from build123d import *

# Parameters (mm, degrees)
F0_R     = 30
F0_R_2   = 6.25
F1_DEPTH = 29
F2_R     = 35
F2_R_2   = 6.25
F3_DEPTH = 6
F4_SIZE  = 3


with BuildPart() as f1:
    # F0 (on Top) → F1 (new body)
    with BuildSketch(Plane.XY):
        Circle(F0_R)
        Circle(F0_R_2, mode=Mode.SUBTRACT)
    extrude(amount=F1_DEPTH)

    # F2 (on Top) → F3 (join)
    with BuildSketch(Plane.XY):
        Circle(F2_R)
        Circle(F2_R_2, mode=Mode.SUBTRACT)
    extrude(amount=F3_DEPTH)

    # F4
    f4_edges = [f1.edges().sort_by_distance(p)[0] for p in [
        (-30, 0, 29),
    ]]
    chamfer(f4_edges, length=F4_SIZE)


solid = f1.part
Read the model definition and answer for the solid it produces. Units are mm, in the model's axes. A direction names the side the tool comes from. Give positions to 0.01 mm unless a question says otherwise; leave off trailing zeros. Write each loop counter-clockwise with the first axis right and the second up, starting at its lowest first coordinate (ties: lowest second). Pieces come first, ordered by that corner, then holes. Notation, with made-up numbers: (-20, -28) -> (8, -28) arc R19 ccw to (8, 1) -> close; hole circle Ø7 at (-3, -8). An arc over 180 degrees is marked (long way). Answer as a JSON object with one key per item and string values. Group by question number.
1) Consider L1, parallel to Y at x = 0, z = 19.25; L2, parallel to Z at x = 25, y = -23.5; L3, parallel to X at y = 5, z = 15.25. Determine where each line is inside the solid, lowest interval first. Write a range as from..to.
2) Find section C-C (z = 27). Write down the section's boundary in (x, y).
3) Find section A-A (x = 0). Write down the section's boundary in (y, z), and give its area (3 significant figures).
4) Each of these flat-tipped pins is pushed along its axis until it touches: P1, Ø1, axis at x = 20.5, z = 20.5, coming from the +Y side; P2, Ø1.5, axis at x = 13.5, y = 26, coming from the +Z side; P3, Ø2, axis at x = 0, z = 17.5, coming from the +Y side; P4, Ø20, axis at x = 0, y = 0, coming from the +Z side. Where does it stop, or does it pass through?
5) A tool of negligible diameter and unlimited length cuts with its end or side. For faces 1 (the cylindrical face through (-29.97, 1.32, 15.86)), 2 (the cylindrical face through (-28, -21, 3)), from which of +Z, -Z, +X, -X, +Y, -Y can it reach the whole face along a straight path? Write none if from no direction.
6) The mould has two halves that part along Y. Classify faces 3 (the cylindrical face through (5.96, 1.88, 14.3)), 4 (the conical face through (-3.534, 26.915, 28.854)), 5 (the flat face through (0, -7, 0)): +Y half, -Y half, draft (parallel to the pull), parting line (faces both ways), or undercut.
7) Find section D-D (z = 18). Write down the section's boundary in (x, y), and give its area (3 significant figures).
Values follow:
{
 "1": {"L1": "y = -30..-6.25, 6.25..30", "L2": "z = 0..6", "L3": "x = -29.58..-3.75, 3.75..29.58"},
 "2": {"outline": "circle Ø58 at (0, 0); hole circle Ø12.5 at (0, 0)"},
 "3": {"outline": "(-35, 0) -> (-6.25, 0) -> (-6.25, 29) -> (-27, 29) -> (-30, 26) -> (-30, 6) -> (-35, 6) -> close; (6.25, 0) -> (35, 0) -> (35, 6) -> (30, 6) -> (30, 26) -> (27, 29) -> (6.25, 29) -> close", "area": "1,430 mm2"},
 "4": {"P1": "stops at y = 22.36", "P2": "stops at z = 27.45", "P3": "stops at y = 30", "P4": "stops at z = 29"},
 "5": {"face 1": "+Z", "face 2": "+Z, -Z"},
 "6": {"face 3": "undercut", "face 4": "parting line", "face 5": "draft"},
 "7": {"outline": "circle Ø60 at (0, 0); hole circle Ø12.5 at (0, 0)", "area": "2,700 mm2"}
}
